Autodesk Inventor part; units mm, degrees
ref_plane "YZ Plane" through (0, 0, 0) normal (1, 0, 0) x (0, 1, 0)
ref_plane "XZ Plane" through (0, 0, 0) normal (0, 1, 0) x (-1, 0, 0)
ref_plane "XY Plane" through (0, 0, 0) normal (0, 0, 1) x (1, 0, 0)
sketch "Sketch1" plane through (0, 0, 0) normal (0, 1, 0) x (-1, 0, 0)
  line L0 (0, 0) -> (60, 0)
  line L1 (60, 0) -> (60, -140)
  line L2 (60, -140) -> (0, -140)
  line L3 (0, -140) -> (0, 0)
  line L4 (30, -20.8594) -> (30, -183.1932) construction
  line L5 (42.5, -21.7206) -> (42.5, -191.0157) construction
  line L6 (17.5, -21.7206) -> (17.5, -184.1979) construction
  circle A0 centre (42.5, -21) radius 1.5
  circle A1 centre (42.5, -41) radius 1.5
  circle A2 centre (42.5, -99) radius 1.5
  circle A3 centre (42.5, -119) radius 1.5
  circle A4 centre (17.5, -99) radius 1.5
  circle A5 centre (17.5, -119) radius 1.5
  circle A6 centre (17.5, -41) radius 1.5
  circle A7 centre (17.5, -21) radius 1.5
  dimension "d0" = 140
  dimension "d1" = 60
  dimension "d2" = 30
  dimension "d3" = 12.5
  dimension "d4" = 12.5
  dimension "d5" = 3
  dimension "d6" = 3
  dimension "d7" = 3
  dimension "d8" = 3
  dimension "d9" = 3
  dimension "d10" = 3
  dimension "d11" = 3
  dimension "d12" = 3
  dimension "d13" = 20
  dimension "d14" = 20
  dimension "d15" = 20
  dimension "d16" = 20
  dimension "d17" = 21
  dimension "d18" = 21
  dimension "d19" = 21
  dimension "d20" = 21
extrude "Extrusion1" add sketch "Sketch1" along normal blind 5
sketch "Sketch2" plane through (0, 0, 0) normal (0, -1, 0) x (1, 0, 0)
  circle A0 centre (-7.5, -20) radius 2.5
  circle A1 centre (-7.5, -120) radius 2.5
  circle A2 centre (-52.5, -20) radius 2.5
  circle A3 centre (-52.5, -120) radius 2.5
  line L0 (-60, 0) -> (0, 0)
  line L1 (0, 0) -> (0, -140)
  line L2 (-60, -140) -> (-60, 0)
  line L3 (0, -140) -> (-60, -140)
  dimension "d23" = 5
  dimension "d24" = 5
  dimension "d25" = 5
  dimension "d26" = 5
  dimension "d27" = 20
  dimension "d28" = 7.5
  dimension "d29" = 20
  dimension "d30" = 7.5
  dimension "d31" = 20
  dimension "d32" = 7.5
  dimension "d33" = 20
  dimension "d34" = 7.5
extrude "Extrusion2" cut sketch "Sketch2" against normal blind 10 contours A0 | A1 | A2 | A3
sketch "Sketch3" plane through (0, 0, 0) normal (0, -1, 0) x (1, 0, 0)
  line L0 (-25, -4) -> (-35, -4)
  line L1 (-35, -4) -> (-35, -9)
  line L2 (-35, -9) -> (-25, -9)
  line L3 (-25, -9) -> (-25, -4)
  line L4 (9.3646, -70) -> (-76.8402, -70) construction
  line L5 (-60, 0) -> (0, 0)
  line L6 (0, 0) -> (0, -140)
  line L7 (-25, -136) -> (-35, -136)
  line L8 (-35, -136) -> (-35, -131)
  line L9 (-35, -131) -> (-25, -131)
  line L10 (-25, -131) -> (-25, -136)
  dimension "d40" = 70
  dimension "d41" = 10
  dimension "d42" = 4
  dimension "d43" = 5
  dimension "d44" = 25
extrude "Extrusion3" cut sketch "Sketch3" against normal blind 10
fillet "Fillet2" radius 5 4 edges at (-60, 2.5, 0) (-60, 2.5, -140) (0, 2.5, -140) (0, 2.5, 0)
sketch "Sketch4" plane through (0, 5, 0) normal (0, 1, 0) x (1, 0, 0)
  circle A0 centre (-50, 76.5) radius 1.5
  circle A1 centre (-50, 93.5) radius 1.5
  circle A2 centre (-20, 76.5) radius 1.5
  circle A3 centre (-10, 93.5) radius 1.5
  line L0 (-5, 140) -> (-55, 140)
  line L1 (-60, 135) -> (-60, 5)
  line L2 (0, 5) -> (0, 135)
  point P0 (0, 0)
  dimension "d49" = 3
  dimension "d50" = 3
  dimension "d51" = 3
  dimension "d52" = 3
  dimension "d53" = 46.5
  dimension "d54" = 46.5
  dimension "d55" = 63.5
  dimension "d56" = 63.5
  dimension "d57" = 10
  dimension "d59" = 10
  dimension "d71" = 10
  dimension "d72" = 20
extrude "Extrusion4" cut sketch "Sketch4" against normal blind 10
sketch "Sketch5" plane through (0, 0, 0) normal (0, -1, 0) x (1, 0, 0)
  line L0 (59.7124, -61) -> (87.7124, -61)
  line L1 (87.7124, -79) -> (59.7124, -79)
  line L2 (5, -61) -> (-15, -61)
  line L3 (-15, -61) -> (-15, -79)
  line L4 (-15, -79) -> (5, -79)
  line L5 (5, -79) -> (5, -61)
  line L6 (0, -5) -> (0, -135)
  point P0 (0, 0)
  dimension "d66" = 15
  dimension "d67" = 5
extrude "Extrusion5" cut sketch "Sketch5" against normal blind 10
fillet "Fillet3" radius 2 4 edges at (0, 2.5, -79) (0, 2.5, -61) (-15, 2.5, -79) (-15, 2.5, -61)
fillet "Fillet4" radius 2 8 edges at (-25, 2.5, -9) (-25, 2.5, -4) (-35, 2.5, -4) (-35, 2.5, -9) (-35, 2.5, -136) (-35, 2.5, -131) (-25, 2.5, -131) (-25, 2.5, -136)
equation "\"d2\" = 0.5 * d1"
equation "\"d4\" = d3"
equation "\"d6\" = d5"
equation "\"d7\" = d5"
equation "\"d8\" = d5"
equation "\"d9\" = d5"
equation "\"d10\" = d5"
equation "\"d11\" = d5"
equation "\"d12\" = d5"
equation "\"d14\" = d13"
equation "\"d15\" = d13"
equation "\"d16\" = d13"
equation "\"d18\" = d17"
equation "\"d19\" = d17"
equation "\"d20\" = d17"
equation "\"d29\" = d27"
equation "\"d30\" = d28"
equation "\"d31\" = d27"
equation "\"d32\" = d28"
equation "\"d33\" = d27"
equation "\"d34\" = d28"
equation "\"d50\" = d49"
equation "\"d51\" = d49"
equation "\"d52\" = d49"
properties part number "Y-Axis_front_plate_bottom"
Read the model definition and answer for the solid it produces. Units are mm, in the model's axes. A direction names the side the tool comes from. Give positions to 0.01 mm unless a question says otherwise; leave off trailing zeros. Loops run counter-clockwise (first coordinate to the right, second up) from the corner with the lowest first, then second, coordinate; pieces in that order, holes last. Notation, with made-up numbers: (64.5, 12.5) - (102.5, 12.5) arc R22 ccw to (102.5, 34.5) - close; hole circle Ø8 at (58.5, 38.5). An arc over 180 degrees is marked (long way). Answer as CSV lines item,"result". Start each with the question number.
1) Determine the mould class of faces 4 (the face through (-59, 3, -2)), 5 (the face through (-15, 2, -70)), 6 (the face through (-60, 2, -69)) for opening direction Z: released by +Z, released by -Z, zero draft, split by the parting line, or undercut.
2) Which of the six approach directions +Z, -Z, +X, -X, +Y, -Y give full straight-line access (tool end or side, diameter ignored) to faces 1 (the face through (-1, 3, -138)), 2 (the face through (-7, 2, -61)), 3 (the face through (-30, 2, -131))?
3) Each of these flat-tipped pins is pushed along its axis until it touches: pin 1 Ø4 at (x, z) = (-20, -76.5) entering from +Y; pin 2 Ø1.8 at (x, z) = (-42.5, -21) entering from +Y. Where does it stop, or does it pass through?
4) Find section B-B (y = 3.5). State how many separate pieces and enclosed holes the cut face has, then the cut area to 3 significant figures.
5) Straight lines are drawn through the part: L1, parallel to Z at x = -17.5, y = 2.95; L2, parallel to X at y = 2.5, z = -18; L3, parallel to Z at x = -12, y = 2.25. For each, find the intervals that lie inside material, in ascending order. Write a range as from..to.
6) Find section A-A (z = -41). Write down the section's boundary in (x, y), then the cut area to 3 significant figures.
Findings below:
1,face 4,"released by +Z"
1,face 5,"undercut"
1,face 6,"zero draft"
2,face 1,"-Z, +X, +Y, -Y"
2,face 2,"+X, +Y, -Y"
2,face 3,"+Y, -Y"
3,pin 1,"y = 5"
3,pin 2,"through"
4,separate pieces,"1"
4,enclosed holes,"18"
4,area,"7,850 mm^2"
5,L1,"-140..-120.5, -117.5..-100.5, -97.5..-42.5, -39.5..-22.5, -19.5..0"
5,L2,"-60..-54, -51..-9, -6..0"
5,L3,"-140..-79, -61..0"
6,outline,"(-60, 0) - (-44, 0) - (-44, 5) - (-60, 5) - close; (-41, 0) - (-19, 0) - (-19, 5) - (-41, 5) - close; (-16, 0) - (0, 0) - (0, 5) - (-16, 5) - close"
6,area,"270 mm^2"
